from build123d import *

# Parameters (mm, degrees)
SKETCH1_W           = 23.2
SKETCH1_H           = 10
BOSS_EXTRUDE1_DEPTH = 20
SKETCH2_W           = 10
SKETCH2_H           = 8.5
BOSS_EXTRUDE2_DEPTH = 3
CHAMFER1_SIZE       = 3
SKETCH3_R           = 2.925
BOSS_EXTRUDE3_DEPTH = 4
BOSS_EXTRUDE4_START = -3.6
SKETCH5_W           = 10
SKETCH5_H           = 32.4
BOSS_EXTRUDE4_DEPTH = 1.25
SKETCH6_R           = 1
CUT_EXTRUDE1_DEPTH  = 1.25
SKETCH7_W           = 10
SKETCH7_H           = 5
BOSS_EXTRUDE5_DEPTH = 12.5
BOSS_EXTRUDE5_TAPER = 5


with BuildPart() as part:
    # Sketch1 → Boss-Extrude1 (new body)
    with BuildSketch(Plane(origin=(0, 0, 0), x_dir=(0, 1, 0), z_dir=(0, 0, 1))):
        with Locations((11.6, 5)):
            Rectangle(SKETCH1_W, SKETCH1_H)
    extrude(amount=BOSS_EXTRUDE1_DEPTH)

    # Sketch2 → Boss-Extrude2 (add)
    with BuildSketch(Plane.XY.offset(20)):
        with Locations((-5, 18.95)):
            Rectangle(SKETCH2_W, SKETCH2_H)
    extrude(amount=BOSS_EXTRUDE2_DEPTH)

    # Chamfer1
    chamfer1_edges = [part.edges().sort_by_distance(p)[0] for p in [
        (-10, 14.7, 21.5),
        (0, 14.7, 21.5),
    ]]
    chamfer(chamfer1_edges, length=CHAMFER1_SIZE)

    # Sketch3 → Boss-Extrude3 (add)
    with BuildSketch(Plane.XY.offset(20)):
        with Locations(Location((-5, 5.2, 0), (0, 0, 180))):
            Circle(SKETCH3_R)
    extrude(amount=BOSS_EXTRUDE3_DEPTH)

    # Sketch5 → Boss-Extrude4 (add)
    with BuildSketch(Plane.XY.offset(20).offset(BOSS_EXTRUDE4_START)):
        with Locations((-5, 11.6)):
            Rectangle(SKETCH5_W, SKETCH5_H)
    extrude(amount=-BOSS_EXTRUDE4_DEPTH)

    # Sketch6 → Cut-Extrude1 (cut)
    with BuildSketch(Plane.XY.offset(16.4)):
        with Locations((-8, -2.7)):
            Circle(SKETCH6_R)
        with Locations((-2, -2.7)):
            Circle(SKETCH6_R)
        with Locations((-8, 25.9)):
            Circle(SKETCH6_R)
        with Locations((-2, 25.9)):
            Circle(SKETCH6_R)
    extrude(amount=-CUT_EXTRUDE1_DEPTH, mode=Mode.SUBTRACT)

    # Sketch7 → Boss-Extrude5 (add)
    with BuildSketch(Plane.XZ):
        with Locations((-5, 2.5)):
            Rectangle(SKETCH7_W, SKETCH7_H)
    extrude(amount=BOSS_EXTRUDE5_DEPTH, taper=BOSS_EXTRUDE5_TAPER)


solid = part.part
Source: CAD feature listing. Evaluate the final solid. Frame: model axes, mm. A direction names the side the tool comes from. Round coordinates to 2 decimals unless told otherwise and drop trailing zeros. Loops run counter-clockwise (first coordinate to the right, second up) from the corner with the lowest first, then second, coordinate; pieces in that order, holes last.
Q1. Mould query, pull axis X, two halves, no side actions, for faces 4 (the face through (-5, 5, 24)), 5 (the face through (-8.13, 26.89, 15.78)), 6 (the face through (-10, 11, 12)). Classes: pulls with the +X half, pulls with the -X half, needs draft (parallel to the pull), parting line crosses it, or undercut.
Q2. Section A-A, the plane z = 21.75. Return loops of the section in (x, y) (3 decimals).
Q3. Ray query, line 1 (Y direction, x = -8, z = 15.9); line 2 (Z direction, x = -3, y = 3); line 3 (Y direction, x = -2, z = 8). Return the intervals inside material, ascending.
Q4. First-contact query: P1, Ø5.5, axis at x = -7, z = 20, coming from the +Y side; P2, Ø1.4, axis at x = -5.5, y = 26.5, coming from the -Z side; P3, Ø1.4, axis at x = -6, y = 25.5, coming from the +Z side. Flat tips, straight axial feed; report the tip coordinate or a pass-through.
Q5. Section B-B, the plane y = 5.2. Return loops of the section in (x, z) (3 decimals), plus the area to 3 significant figures.
Q6. Section D-D, the plane z = 10. Return loops of the section in (x, y).
Q7. Section C-C, the plane y = -2.7. State how many separate pieces and enclosed holes the cut face has, plus the area to 3 significant figures.
Q8. Access query for faces 1 (the face through (-5, -4.6, 16)), 2 (the face through (-1.5, 16.2, 21.5)), 3 (the face through (-5, 9, 20)). Directions: +Z, -Z, +X, -X, +Y, -Y. A direction counts if a zero-diameter tool reaches every point of the face in a straight line with its end or side. Return the directions, or none.
Solutions:
1. face 4: needs draft
1. face 5: undercut
1. face 6: pulls with the -X half
2. outline: (-10, 17.7) - (-7, 14.7) - (-3, 14.7) - (0, 17.7) - (0, 23.2) - (-10, 23.2) - close; circle Ø5.85 at (-5, 5.2)
3. line 1: y = -4.6 to -3.7, -1.7 to 24.9, 26.9 to 27.8
3. line 2: z = 0 to 20
3. line 3: y = 0 to 23.2
4. P1: stops at y = 23.2
4. P2: stops at z = 15.15
4. P3: stops at z = 16.4
5. outline: (-10, 0) - (0, 0) - (0, 20) - (-2.075, 20) - (-2.075, 24) - (-7.925, 24) - (-7.925, 20) - (-10, 20) - close
5. area: 223 mm2
6. outline: (-10, 0) - (0, 0) - (0, 23.2) - (-10, 23.2) - close
7. separate pieces: 4
7. enclosed holes: 0
7. area: 50.6 mm2
8. face 1: +Z, +X, -X, -Y
8. face 2: +Z, +X
8. face 3: +Z
